from build123d import *

# Parameters (mm, degrees)
SKETCH_W        = 25
SKETCH_H        = 54
PAD_DEPTH       = 32
SKETCH001_W     = 15.2
SKETCH001_H     = 15.2
SKETCH001_W_2   = 18
SKETCH001_H_2   = 18
POCKET_DEPTH    = 32.001
SKETCH002_W     = 20.2
SKETCH002_H     = 20.2
POCKET001_DEPTH = 30
SKETCH005_W     = 2.8
SKETCH005_H     = 5.7
POCKET002_DEPTH = 6
SKETCH003_R     = 1.7
POCKET003_DEPTH = 6
SKETCH006_W     = 5.7
SKETCH006_H     = 2.8
POCKET004_DEPTH = 6
SKETCH004_R     = 1.7
POCKET005_DEPTH = 6
SKETCH007_W     = 4
SKETCH007_H     = 13
POCKET006_DEPTH = 10
FILLET_R        = 2
SKETCH008_R     = 0.632456
SKETCH008_R_2   = 0.6
POCKET007_DEPTH = 32.001


with BuildPart() as part:
    # Sketch → Pad (new body)
    with BuildSketch(Plane.XY):
        with Locations((0, -2)):
            Rectangle(SKETCH_W, SKETCH_H)
    extrude(amount=PAD_DEPTH)

    # Sketch001 → Pocket (cut, through all)
    with BuildSketch(Plane(origin=(0, 0, 0), x_dir=(1, 0, 0), z_dir=(0, 0, -1))):
        with Locations((0, 16.6)):
            Rectangle(SKETCH001_W, SKETCH001_H)
        with Locations((0, -9.982677)):
            Rectangle(SKETCH001_W_2, SKETCH001_H_2)
    extrude(amount=-POCKET_DEPTH, mode=Mode.SUBTRACT)

    # Sketch002 → Pocket001 (cut)
    with BuildSketch(Plane.XY.offset(32)):
        with Locations((0, 10.1)):
            Rectangle(SKETCH002_W, SKETCH002_H)
    extrude(amount=-POCKET001_DEPTH, mode=Mode.SUBTRACT)

    # Sketch005 → Pocket002 (cut)
    with BuildSketch(Plane.XY.offset(32)):
        with Locations((9.935363, -7.131511)):
            Rectangle(SKETCH005_W, SKETCH005_H)
        with Locations((9.987245, -16.468893)):
            Rectangle(SKETCH005_W, SKETCH005_H)
    extrude(amount=-POCKET002_DEPTH, mode=Mode.SUBTRACT)

    # Sketch003 → Pocket003 (cut)
    with BuildSketch(Plane.YZ.offset(12.5)):
        with Locations((-6.998034, 28.990236)):
            Circle(SKETCH003_R)
        with Locations((-16.503597, 29.011274)):
            Circle(SKETCH003_R)
    extrude(amount=-POCKET003_DEPTH, mode=Mode.SUBTRACT)

    # Sketch006 → Pocket004 (cut)
    with BuildSketch(Plane(origin=(0, 0, 0), x_dir=(-1, 0, 0), z_dir=(0, 1, 0))):
        with Locations((0, 28.604247)):
            Rectangle(SKETCH006_W, SKETCH006_H)
    extrude(amount=-POCKET004_DEPTH, mode=Mode.SUBTRACT)

    # Sketch004 → Pocket005 (cut)
    with BuildSketch(Plane.XY.offset(32)):
        with Locations((0, -3)):
            Circle(SKETCH004_R)
    extrude(amount=-POCKET005_DEPTH, mode=Mode.SUBTRACT)

    # Sketch007 → Pocket006 (cut)
    with BuildSketch(Plane.XY.offset(32)):
        with Locations((-11, 10.1)):
            Rectangle(SKETCH007_W, SKETCH007_H)
    extrude(amount=-POCKET006_DEPTH, mode=Mode.SUBTRACT)

    # Fillet
    fillet_edges = [part.edges().sort_by_distance(p)[0] for p in [
        (12.5, -2, 0),
        (0, -29, 0),
        (-12.5, -2, 0),
        (0, 25, 0),
    ]]
    fillet(fillet_edges, radius=FILLET_R)

    # Sketch008 → Pocket007 (cut, through all)
    with BuildSketch(Plane(origin=(0, 0, 0), x_dir=(1, 0, 0), z_dir=(0, 0, -1))):
        with Locations((-7.6, 24.200001)):
            Circle(SKETCH008_R)
        with Locations((7.6, 24.2)):
            Circle(SKETCH008_R)
        with Locations((7.6, 9)):
            Circle(SKETCH008_R_2)
        with Locations((-7.6, 9)):
            Circle(SKETCH008_R_2)
    extrude(amount=-POCKET007_DEPTH, mode=Mode.SUBTRACT)


solid = part.part
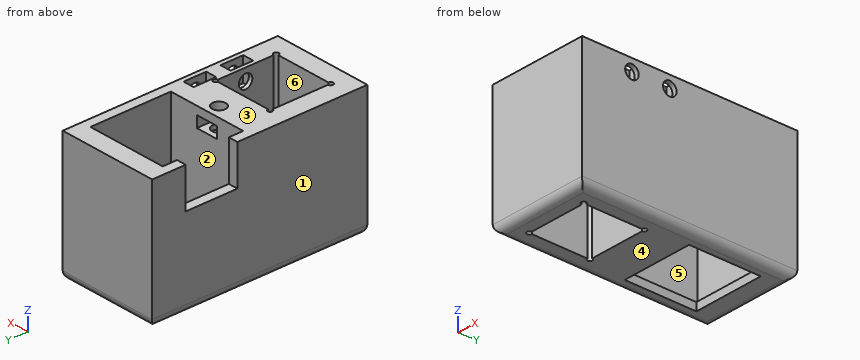
CAD build for the part. Positions are in the model's coordinates, mm. Face numbers are marked on the shaded views. A direction names the side the tool comes from. Give positions to 0.01 mm unless a question says otherwise; leave off trailing zeros. Order: outer loops, then holes, each group sorted by start corner. A loop starts at its lowest first (then second) coordinate and runs counter-clockwise, first axis right, second up. Notation, with made-up numbers: (9, 18.25) - (32, 18.25) arc R23 cw to (32, 29.25) - close; hole circle Ø8 at (55.25, 79.25). An arc over 180 degrees is marked (long way). Write each question's results on one line, items separated by ' | '.
1. Saw through at C-C on y = -2. List the corners of the cut face in (x, z).
Calculated:
outline: (-12.5, 2) arc R2 ccw to (-10.5, 0) - (10.5, 0) arc R2 ccw to (12.5, 2) - (12.5, 32) - (1.37, 32) - (1.37, 30) - (2.85, 30) - (2.85, 27.2) - (1.37, 27.2) - (1.37, 26) - (-1.37, 26) - (-1.37, 27.2) - (-2.85, 27.2) - (-2.85, 30) - (-1.37, 30) - (-1.37, 32) - (-12.5, 32) - close
2. Saw through at B-B on z = 4.5. List the corners of the cut face in (x, y), and give its area (3 significant figures).
Calculated:
outline: (-12.5, -29) - (12.5, -29) - (12.5, 25) - (-12.5, 25) - close; hole (-10.1, 0) - (10.1, 0) - (10.1, 20.2) - (-10.1, 20.2) - close; hole (-7.6, -23.57) arc R0.63 ccw (long way) to (-6.97, -24.2) - (6.97, -24.2) arc R0.63 ccw (long way) to (7.6, -23.57) - (7.6, -9.6) arc R0.6 ccw (long way) to (7, -9) - (-7, -9) arc R0.6 ccw (long way) to (-7.6, -9.6) - close | area: 707 mm2
3. Probe L1, parallel to Y at x = 1, z = 7; L2, parallel to Y at x = 0, z = 30.6; L3, parallel to X at y = -13, z = 31. List the from-to ranges inside material, lowest first. Write a range as from..to.
Calculated:
L1: y = -29..-24.2, -9..0, 20.2..25 | L2: y = -29..-24.2, -9..-4.7, -1.3..0, 20.2..25 | L3: x = -12.5..-7.6, 7.6..12.5
4. Pull direction X, two halves, no side cores. Call the marked faces 1, 2 and 3: released by +X, released by -X, zero draft, split by the parting line, or undercut.
Calculated:
face 1: released by -X | face 2: undercut | face 3: zero draft
5. 3-axis set-ups, long thin cutter, end or side, ignore diameter. For the marked faces 4, 5 and 6: which of +Z, -Z, +X, -X, +Y, -Y reach the whole face in a straight line?
Calculated:
face 4: -Z, +X, -X, +Y, -Y | face 5: +Z | face 6: +Z, -Z
6. Pin check, flat tip, straight feed: pin 1 (1 mm diameter, centred on x = 0, y = -23, fed in from +Z). Stop position of the tip, or through.
Calculated:
pin 1: passes through
7. Saw through at A-A on y = -21.5. List the corners of the cut face in (x, z).
Calculated:
outline: (-12.5, 2) arc R2 ccw to (-10.5, 0) - (-7.6, 0) - (-7.6, 32) - (-12.5, 32) - close; (7.6, 0) - (10.5, 0) arc R2 ccw to (12.5, 2) - (12.5, 32) - (7.6, 32) - close
